Check sheet for the modelled part. Datum: model origin and axes. Units: mm. A direction names the side the tool comes from. Give positions to 0.01 mm unless a question says otherwise; leave off trailing zeros. Loops run counter-clockwise (first coordinate to the right, second up) from the corner with the lowest first, then second, coordinate; pieces in that order, holes last. Notation, with made-up numbers: (74.5, -9.75) -> (82.5, -9.75) arc R27 ccw to (82.5, 18.25) -> close; hole circle Ø4 at (4.5, 86). An arc over 180 degrees is marked (long way). Write each question's results on one line, items separated by ' | '. Start each with the question number.
1. Cross-section at D-D on x = -7. Record the boundary of the cut face in (y, z).
2. Cross-section at C-C on x = 0. Record the boundary of the cut face in (y, z).
3. Material ranges on L1, parallel to X at y = 1.15, z = 0 (3 decimals); L2, parallel to X at y = 3.4, z = 0 (3 decimals); L3, parallel to Z at x = 16, y = 11.75, recorded low to high. Write a range as from..to.
4. Tool access check on faces 1 (the face through (1.198, 3.32, 3.804)), 2 (the face through (-17.145, 4, 1)), 3 (the face through (-8, 9, -5.131)). Record the directions out of +Z, -Z, +X, -X, +Y, -Y that give a thin tool (end or side, any length) a straight path to the whole face; none if there is none.
5. Gauge pin test, flat ends, axial feed: pin 1 Ø3 at (x, z) = (3, 0) entering from +Y; pin 2 Ø3 at (x, z) = (2.5, 4) entering from +Y; pin 3 Ø2 at (x, z) = (0, 0) entering from +Y. Record the tip position at first contact, or that the pin passes through.
6. Cross-section at B-B on y = 8.25. Record the boundary of the cut face in (x, z) (3 decimals).
7. Mould release check, pull along Z, two halves, no side actions. Record for faces 4 (the face through (0, 4, 5.842)), 5 (the face through (-1.76, 1.03, -0.39)), 6 (the face through (17.145, 4, 1)): +Z half, -Z half, draft (parallel to the pull), parting line (faces both ways), or undercut.
8. Cross-section at A-A on z = 0. Record the boundary of the cut face in (x, y) (3 decimals).
from build123d import *

# Parameters (mm, degrees)
SKETCH1_W           = 34.29
SKETCH1_H           = 11.684
BOSS_EXTRUDE1_DEPTH = 13.462
SKETCH3_W           = 15.494
SKETCH3_H           = 8.636
CUT_EXTRUDE1_DEPTH  = 23.622
SKETCH4_W           = 34.29
SKETCH4_H           = 10.2616
CUT_EXTRUDE2_DEPTH  = 8.89
SKETCH5_R           = 3.9878
CUT_EXTRUDE3_DEPTH  = 2.54
SKETCH6_R           = 1.8034
CUT_EXTRUDE4_DEPTH  = 7.62


with BuildPart() as part:
    # Sketch1 → Boss-Extrude1 (new body)
    with BuildSketch(Plane(origin=(0, 0, 0), x_dir=(1, 0, 0), z_dir=(0, 1, 0))):
        Rectangle(SKETCH1_W, SKETCH1_H)
    extrude(amount=BOSS_EXTRUDE1_DEPTH)

    # Sketch3 → Cut-Extrude1 (cut)
    with BuildSketch(Plane.XY.offset(5.842)):
        with Locations((0, 9.144)):
            Rectangle(SKETCH3_W, SKETCH3_H)
    extrude(amount=-CUT_EXTRUDE1_DEPTH, mode=Mode.SUBTRACT)

    # Sketch4 → Cut-Extrude2 (cut)
    with BuildSketch(Plane(origin=(0, 13.462, 0), x_dir=(1, 0, 0), z_dir=(0, 1, 0))):
        Rectangle(SKETCH4_W, SKETCH4_H)
    extrude(amount=-CUT_EXTRUDE2_DEPTH, mode=Mode.SUBTRACT)

    # Sketch5 → Cut-Extrude3 (cut)
    with BuildSketch(Plane(origin=(0, 4.572, 0), x_dir=(1, 0, 0), z_dir=(0, 1, 0))):
        with Locations(Location((0, 0, 0), (0, 0, 270))):
            Circle(SKETCH5_R)
    extrude(amount=-CUT_EXTRUDE3_DEPTH, mode=Mode.SUBTRACT)

    # Sketch6 → Cut-Extrude4 (cut)
    with BuildSketch(Plane(origin=(0, 2.032, 0), x_dir=(1, 0, 0), z_dir=(0, 1, 0))):
        with Locations(Location((0, 0, 0), (0, 0, 270))):
            Circle(SKETCH6_R)
    extrude(amount=-CUT_EXTRUDE4_DEPTH, mode=Mode.SUBTRACT)


solid = part.part
Geometry says:
1) outline: (0, -5.84) -> (4.83, -5.84) -> (4.83, -5.13) -> (4.57, -5.13) -> (4.57, 5.13) -> (4.83, 5.13) -> (4.83, 5.84) -> (0, 5.84) -> close
2) outline: (0, -5.84) -> (4.83, -5.84) -> (4.83, -5.13) -> (4.57, -5.13) -> (4.57, -3.99) -> (2.03, -3.99) -> (2.03, -1.8) -> (0, -1.8) -> close; (0, 1.8) -> (2.03, 1.8) -> (2.03, 3.99) -> (4.57, 3.99) -> (4.57, 5.13) -> (4.83, 5.13) -> (4.83, 5.84) -> (0, 5.84) -> close
3) L1: -17.145..-1.803, 1.803..17.145 | L2: -17.145..-3.988, 3.988..17.145 | L3: -5.84..-5.13, 5.13..5.84
4) face 1: +Y | face 2: +Z, -Z, -X, +Y, -Y | face 3: +X, -X, +Y
5) pin 1: y = 4.57 | pin 2: y = 4.83 | pin 3: through
6) outline: (-17.145, -5.842) -> (-7.747, -5.842) -> (-7.747, -5.131) -> (-17.145, -5.131) -> close; (-17.145, 5.131) -> (-7.747, 5.131) -> (-7.747, 5.842) -> (-17.145, 5.842) -> close; (7.747, -5.842) -> (17.145, -5.842) -> (17.145, -5.131) -> (7.747, -5.131) -> close; (7.747, 5.131) -> (17.145, 5.131) -> (17.145, 5.842) -> (7.747, 5.842) -> close
7) face 4: +Z half | face 5: undercut | face 6: draft
8) outline: (-17.145, 0) -> (-1.803, 0) -> (-1.803, 2.032) -> (-3.988, 2.032) -> (-3.988, 4.572) -> (-17.145, 4.572) -> close; (1.803, 0) -> (17.145, 0) -> (17.145, 4.572) -> (3.988, 4.572) -> (3.988, 2.032) -> (1.803, 2.032) -> close
